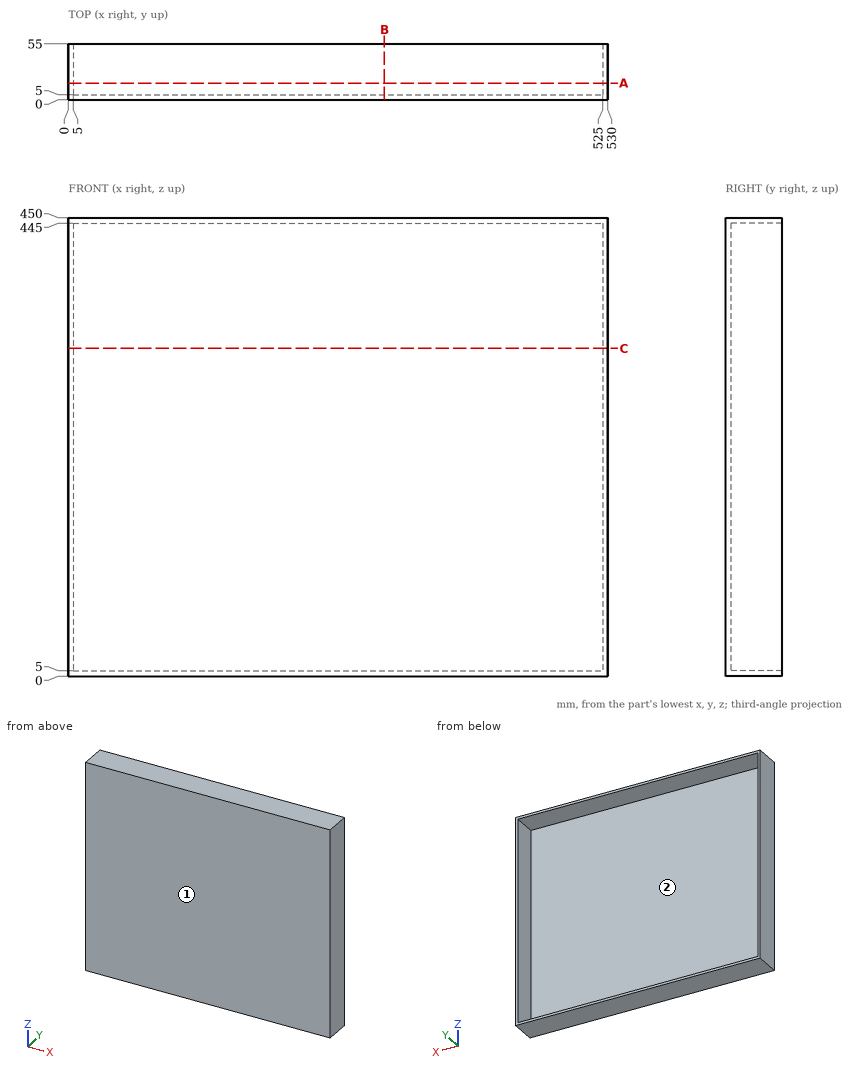
Check sheet for the drawn part. Datum: minimum x, y, z corner. Units: mm. Round coordinates to 2 decimals unless told otherwise and drop trailing zeros. Loops run counter-clockwise (first coordinate to the right, second up) from the corner with the lowest first, then second, coordinate; pieces in that order, holes last.
Item 1: Cross-section at A-A on y = 16.5. Record the boundary of the cut face in (x, z), then the cut area to 3 significant figures.
Item 2: Cross-section at C-C on z = 322. Record the boundary of the cut face in (x, y).
Item 3: Mould release check, pull along X, two halves, no side actions. Record for the marked faces 1 and 2: pulls with the +X half, pulls with the -X half, needs draft (parallel to the pull), parting line crosses it, or undercut.
Item 4: Cross-section at B-B on x = 310.5. Record the boundary of the cut face in (y, z), then the cut area to 3 significant figures.
Item 5: Gauge pin test, flat end, axial feed: pin 1 (6 mm diameter, centred on x = 195.5, z = 294, fed in from +Y). Record the tip position at first contact, or that the pin passes through.
Item 6: Thickness scan on line 1 (Z direction, x = 101.5, y = 9.5); line 2 (X direction, y = 37, z = 341.5); line 3 (Y direction, x = 324, z = 286.5). Record the ranges inside material, lowest first.
Answer sheet:
1. outline: (0, 0) - (530, 0) - (530, 450) - (0, 450) - close; hole (5, 5) - (525, 5) - (525, 445) - (5, 445) - close
1. area: 9,700 mm2
2. outline: (0, 0) - (530, 0) - (530, 55) - (525, 55) - (525, 5) - (5, 5) - (5, 55) - (0, 55) - close
3. face 1: needs draft
3. face 2: undercut
4. outline: (0, 0) - (55, 0) - (55, 5) - (5, 5) - (5, 445) - (55, 445) - (55, 450) - (0, 450) - close
4. area: 2,750 mm2
5. pin 1: stops at y = 5
6. line 1: z = 0 to 5, 445 to 450
6. line 2: x = 0 to 5, 525 to 530
6. line 3: y = 0 to 5
